Read the model definition and answer for the solid it produces. Units are mm, in the model's axes. A direction names the side the tool comes from. Round coordinates to 2 decimals unless told otherwise and drop trailing zeros. Loops run counter-clockwise (first coordinate to the right, second up) from the corner with the lowest first, then second, coordinate; pieces in that order, holes last. Notation, with made-up numbers: M 36.5,-29 L 57.5,-29 A16 cw 57.5,-9 Z; hole C 83,-7 d2. An arc over 180 degrees is marked long. Write each question's results on one line, items separated by ' | '.
```python
from build123d import *

# Parameters (mm, degrees)
SKETCH2_R           = 8
SKETCH2_R_2         = 3.25
BOSS_EXTRUDE1_DEPTH = 7.5
SKETCH3_R           = 6
CUT_EXTRUDE1_DEPTH  = 3.775
SKETCH4_R           = 0.8
CUT_EXTRUDE2_DEPTH  = 10


with BuildPart() as part:
    # Sketch2 → Boss-Extrude1 (new body)
    with BuildSketch(Plane(origin=(0, 0, 0), x_dir=(0, 0, -1), z_dir=(1, 0, 0))):
        Circle(SKETCH2_R)
        Circle(SKETCH2_R_2, mode=Mode.SUBTRACT)
    extrude(amount=BOSS_EXTRUDE1_DEPTH)

    # Sketch3 → Cut-Extrude1 (cut)
    with BuildSketch(Plane(origin=(7.5, 0, 0), x_dir=(0, 0, -1), z_dir=(1, 0, 0))):
        Circle(SKETCH3_R)
    extrude(amount=-CUT_EXTRUDE1_DEPTH, mode=Mode.SUBTRACT)

    # Sketch4 → Cut-Extrude2 (cut)
    with BuildSketch(Plane(origin=(7.5, 0, 0), x_dir=(0, 0, -1), z_dir=(1, 0, 0))):
        with Locations((0, 7.9)):
            Circle(SKETCH4_R)
    extrude(amount=-CUT_EXTRUDE2_DEPTH, mode=Mode.SUBTRACT)


solid = part.part
```
1. Which of the six approach directions +Z, -Z, +X, -X, +Y, -Y give full straight-line access (tool end or side, diameter ignored) to faces 1 (the face through (7.5, -2, 6)), 2 (the face through (3.725, -3, -3))?
Completed:
face 1: +Z, -Z, +X, +Y, -Y | face 2: +X
2. Find the intervals of material crossed by L1, parallel to Z at x = 1.5, y = 0; L2, parallel to Y at x = 4.6, z = 0; L3, parallel to X at y = 3.75, z = 4.5 (3 decimals), in increasing order.
Completed:
L1: z = -8 to -3.25, 3.25 to 8 | L2: y = -8 to -6, 6 to 7.1 | L3: x = 0 to 3.725
3. Find section B-B, the plane z = -1.5. Give the vertices of the cut face in (x, y) (3 decimals).
Completed:
outline: M 0,-7.858 L 7.5,-7.858 L 7.5,-5.809 L 3.725,-5.809 L 3.725,-2.883 L 0,-2.883 Z; M 0,2.883 L 3.725,2.883 L 3.725,5.809 L 7.5,5.809 L 7.5,7.858 L 0,7.858 Z
4. Find section C-C, the plane z = 4.25. Give the vertices of the cut face in (x, y) (3 decimals).
Completed:
outline: M 0,-6.778 L 7.5,-6.778 L 7.5,-4.235 L 3.725,-4.235 L 3.725,4.235 L 7.5,4.235 L 7.5,6.778 L 0,6.778 Z
5. Given P1, Ø9.5, axis at y = 0, z = 0, coming from the +X side (3 decimals), flat-ended and moving along its own axis, determine where the tip first touches the part or whether it passes through.
Completed:
P1: stops at x = 3.725
6. Find section D-D, the plane y = -5.75. Give the vertices of the cut face in (x, z) (3 decimals), then the cut area to 3 significant figures.
Completed:
outline: M 0,-5.562 L 7.5,-5.562 L 7.5,-1.714 L 3.725,-1.714 L 3.725,1.714 L 7.5,1.714 L 7.5,5.562 L 0,5.562 Z | area: 70.5 mm2
7. Find section A-A, the plane y = 0. Give the vertices of the cut face in (x, z) (3 decimals), then the cut area to 3 significant figures.
Completed:
outline: M 0,-8 L 7.5,-8 L 7.5,-6 L 3.725,-6 L 3.725,-3.25 L 0,-3.25 Z; M 0,3.25 L 3.725,3.25 L 3.725,6 L 7.5,6 L 7.5,8 L 0,8 Z | area: 50.5 mm2
8. Determine the mould class of faces 3 (the face through (0, 0.1, -3.4)), 4 (the face through (4, -8, 0)), 5 (the face through (1.836, -1.978, 2.579)) for opening direction Y: released by +Y, released by -Y, zero draft, split by the parting line, or undercut.
Completed:
face 3: zero draft | face 4: split by the parting line | face 5: undercut
